```python
from build123d import *

# Parameters (mm, degrees)
BOSS_EXTRUDE1_DEPTH = 1.27
FILLET1_START       = -1
FILLET1_DEPTH       = 3
FILLET2_START       = -1
FILLET2_DEPTH       = 3
FILLET3_R           = 5.08
FILLET4_R           = 5.08
SKETCH3_R           = 1.27
CUT_EXTRUDE1_DEPTH  = 39.269062151


with BuildPart() as part:
    # Sketch1 → Boss-Extrude1 (new body)
    with BuildSketch(Plane.XY):
        with BuildLine():
            add(Edge.make_bspline(
                [(-26.078451224, -26.078451224), (-25.595030672, -26.46689269), (-16.201372292, -29.50543677), (0, -7.636650328), (16.201372291, -29.50543677), (25.595030672, -26.46689269), (26.078451224, -26.078451224)],
                knots=[0.032766754, 0.032766754, 0.032766754, 0.032766754, 0.065533508, 0.5, 0.934466492, 0.967233246, 0.967233246, 0.967233246, 0.967233246], degree=3))
            add(Edge.make_bspline(
                [(26.078451224, -26.078451224), (26.46689269, -25.595030672), (29.505436772, -16.201372289), (7.636650328, -2e-09), (29.505436768, 16.201372294), (26.46689269, 25.595030672), (26.078451224, 26.078451224)],
                knots=[0.032766754, 0.032766754, 0.032766754, 0.032766754, 0.065533508, 0.5, 0.934466492, 0.967233246, 0.967233246, 0.967233246, 0.967233246], degree=3))
            add(Edge.make_bspline(
                [(-26.078451224, 26.078451224), (-25.595030672, 26.46689269), (-16.201372292, 29.50543677), (0, 7.636650328), (16.201372291, 29.50543677), (25.595030672, 26.46689269), (26.078451224, 26.078451224)],
                knots=[0.032766754, 0.032766754, 0.032766754, 0.032766754, 0.065533508, 0.5, 0.934466492, 0.967233246, 0.967233246, 0.967233246, 0.967233246], degree=3))
            add(Edge.make_bspline(
                [(-26.078451224, -26.078451224), (-26.46689269, -25.595030672), (-29.50543677, -16.201372292), (-7.636650328, 0), (-29.50543677, 16.201372291), (-26.46689269, 25.595030672), (-26.078451224, 26.078451224)],
                knots=[0.032766754, 0.032766754, 0.032766754, 0.032766754, 0.065533508, 0.5, 0.934466492, 0.967233246, 0.967233246, 0.967233246, 0.967233246], degree=3))
        make_face()
    extrude(amount=BOSS_EXTRUDE1_DEPTH)

    # Fillet1: read off the stored shape, not the designer's step
    # Fillet1 outline → Fillet1 (cut)
    with BuildSketch(Plane.XY.offset(FILLET1_START)):
        with BuildLine():
            add(Edge.make_bspline(
                [(26.078451224, 26.078451224), (25.595030672, 26.46689269), (24.088787806, 26.954113447), (22.608220096, 27.071858625), (21.782533291, 27.042115453)],
                knots=[0.032766754, 0.032766754, 0.032766754, 0.032766754, 0.065533508, 0.1076861, 0.1076861, 0.1076861, 0.1076861], degree=3))
            ThreePointArc((21.782533291, 27.042115453), (25.557510624, 25.557510623), (27.042115452, 21.78253329))
            add(Edge.make_bspline(
                [(27.042115452, 21.78253329), (27.071858625, 22.608220095), (26.954113447, 24.088787806), (26.46689269, 25.595030672), (26.078451224, 26.078451224)],
                knots=[0.8923139, 0.8923139, 0.8923139, 0.8923139, 0.934466492, 0.967233246, 0.967233246, 0.967233246, 0.967233246], degree=3))
        make_face()
    extrude(amount=FILLET1_DEPTH, mode=Mode.SUBTRACT)

    # Fillet2: read off the stored shape, not the designer's step
    # Fillet2 outline → Fillet2 (cut)
    with BuildSketch(Plane.XY.offset(FILLET2_START)):
        with BuildLine():
            add(Edge.make_bspline(
                [(-26.078451224, -26.078451224), (-25.595030672, -26.46689269), (-24.088787806, -26.954113447), (-22.608220096, -27.071858625), (-21.782533291, -27.042115453)],
                knots=[0.032766754, 0.032766754, 0.032766754, 0.032766754, 0.065533508, 0.1076861, 0.1076861, 0.1076861, 0.1076861], degree=3))
            ThreePointArc((-21.782533291, -27.042115453), (-25.557510624, -25.557510624), (-27.042115453, -21.782533291))
            add(Edge.make_bspline(
                [(-27.042115453, -21.782533291), (-27.071858625, -22.608220096), (-26.954113447, -24.088787806), (-26.46689269, -25.595030672), (-26.078451224, -26.078451224)],
                knots=[0.8923139, 0.8923139, 0.8923139, 0.8923139, 0.934466492, 0.967233246, 0.967233246, 0.967233246, 0.967233246], degree=3))
        make_face()
    extrude(amount=FILLET2_DEPTH, mode=Mode.SUBTRACT)

    # Fillet3
    fillet3_edges = [part.edges().sort_by_distance(p)[0] for p in [
        (-26.078451224, 26.078451224, 0.635),
    ]]
    fillet(fillet3_edges, radius=FILLET3_R)

    # Fillet4
    fillet4_edges = [part.edges().sort_by_distance(p)[0] for p in [
        (26.078451224, -26.078451224, 0.635),
    ]]
    fillet(fillet4_edges, radius=FILLET4_R)

    # Sketch3 → Cut-Extrude1 (cut, through all)
    with BuildSketch(Plane.XY.offset(1.27)):
        with Locations((-22.483919179, 22.563317918)):
            Circle(SKETCH3_R)
        with Locations((-22.351271412, -22.337766752)):
            Circle(SKETCH3_R)
        with Locations((22.549813258, -22.205118985)):
            Circle(SKETCH3_R)
        with Locations((22.418317518, 22.306006297)):
            Circle(SKETCH3_R)
        with BuildLine():
            add(Edge.make_bspline(
                [(-7.336925612, -7.336925612), (-7.094564954, -7.539990493), (-4.441685448, -8.467510629), (0, -2.70941912), (4.441685448, -8.467510629), (7.094564954, -7.539990493), (7.336925612, -7.336925612)],
                knots=[0.055321023, 0.055321023, 0.055321023, 0.055321023, 0.110642047, 0.5, 0.889357953, 0.944678976, 0.944678976, 0.944678976, 0.944678976], degree=3))
            add(Edge.make_bspline(
                [(7.336925612, 7.336925612), (7.539990493, 7.094564954), (8.467510629, 4.441685448), (2.70941912, 0), (8.467510629, -4.441685448), (7.539990493, -7.094564954), (7.336925612, -7.336925612)],
                knots=[0.055321023, 0.055321023, 0.055321023, 0.055321023, 0.110642047, 0.5, 0.889357953, 0.944678977, 0.944678977, 0.944678977, 0.944678977], degree=3))
            add(Edge.make_bspline(
                [(-7.336925612, 7.336925612), (-7.094564954, 7.539990493), (-4.441685448, 8.467510629), (0, 2.70941912), (4.441685448, 8.467510629), (7.094564954, 7.539990493), (7.336925612, 7.336925612)],
                knots=[0.055321023, 0.055321023, 0.055321023, 0.055321023, 0.110642047, 0.5, 0.889357953, 0.944678977, 0.944678977, 0.944678977, 0.944678977], degree=3))
            add(Edge.make_bspline(
                [(-7.336925612, 7.336925612), (-7.539990493, 7.094564954), (-8.467510629, 4.441685448), (-2.70941912, 0), (-8.467510629, -4.441685448), (-7.539990493, -7.094564954), (-7.336925612, -7.336925612)],
                knots=[0.055321023, 0.055321023, 0.055321023, 0.055321023, 0.110642047, 0.5, 0.889357953, 0.944678977, 0.944678977, 0.944678977, 0.944678977], degree=3))
        make_face()
    extrude(amount=-CUT_EXTRUDE1_DEPTH, mode=Mode.SUBTRACT)


solid = part.part
```
Part model, mm, in its own coordinate system. Round coordinates to 2 decimals unless told otherwise and drop trailing zeros. Put each result on its own line as item: value. Start each with the question number.
1. Drill centre lines: probe 1 along Y at (x, z) = (6, 1.1); probe 2 along X at (y, z) = (22, 0.2); probe 3 along X at (y, z) = (-22, 1.15). Where is each one in solid material? Low to high. Write a range as [from, to].
2. Slice it at A-A on z = 0.5. State how many separate pieces and enclosed holes the cut face has, then the cut area to 3 significant figures.
3. Two-plate mould, pull along X, no slides. Class faces 1 (the face through (0, -6, 1.27)), 2 (the face through (-23.62, -22.28, 0.64)): +X half, -X half, draft (parallel to the pull), parting line (faces both ways), or undercut.
4. Drop a flat-ended pin along its axis: pin 1 (2 mm diameter, centred on x = -22.48, y = 22.56, fed in from -Z). Give the stop position or say it passes through.
Findings:
1. probe 1: [-19.86, -7.75], [-1.93, 1.93], [7.75, 19.86]
1. probe 2: [-27.05, -23.62], [-21.35, -9.82], [9.82, 21.19], [23.65, 27.05]
1. probe 3: [-27.05, -23.58], [-21.13, -9.82], [9.82, 21.3], [23.8, 27.05]
2. separate pieces: 1
2. enclosed holes: 5
2. area: 1,930 mm2
3. face 1: draft
3. face 2: undercut
4. pin 1: through
